The model under review builds one solid part; all positions refer to its coordinate system, in mm. A direction names the side the tool comes from. Give positions to 0.01 mm unless a question says otherwise; leave off trailing zeros. Order: outer loops, then holes, each group sorted by start corner. A loop starts at its lowest first (then second) coordinate and runs counter-clockwise, first axis right, second up. Notation, with made-up numbers: (19, 28.5) -> (34, 28.5) arc R30 ccw to (34, 52.5) -> close; hole circle Ø7 at (61.25, 61). An arc over 180 degrees is marked (long way). Answer as a JSON object with one key per item and string values. Group by question number.
from build123d import *

# Parameters (mm, degrees)
F0_R      = 55
F1_DEPTH  = 4
F2_R      = 22.1
F3_DEPTH  = 2
F4_R      = 25.3
F4_R_2    = 22.1
F5_DEPTH  = 1.5
F6_R      = 25.3
F6_R_2    = 23.5
F7_DEPTH  = 1.5
F8_DEPTH  = 0.2
F9_R      = 28
F9_R_2    = 25.3
F10_DEPTH = 1
F11_R     = 5
F12_DEPTH = 25
F14_DEPTH = 1
F15_R     = 1.45
F16_DEPTH = 25
F17_R     = 1.45
F18_DEPTH = 25


with BuildPart() as f1:
    # F0 (on Top) → F1 (new body)
    with BuildSketch(Plane.XY):
        Circle(F0_R)
    extrude(amount=F1_DEPTH)

    # F2 (on face) → F3 (cut)
    with BuildSketch(Plane.XY.offset(4)):
        with Locations((27, 0)):
            Circle(F2_R)
    extrude(amount=-F3_DEPTH, mode=Mode.SUBTRACT)

    # F4 (on face) → F5 (cut)
    with BuildSketch(Plane.XY.offset(4)):
        with Locations((27, 0)):
            Circle(F4_R)
        with Locations((27, 0)):
            Circle(F4_R_2, mode=Mode.SUBTRACT)
    extrude(amount=-F5_DEPTH, mode=Mode.SUBTRACT)

    # F6 (on face) → F7 (cut)
    with BuildSketch(Plane.XY.offset(2.5)):
        with Locations((27, 0)):
            Circle(F6_R)
        with Locations((27, 0)):
            Circle(F6_R_2, mode=Mode.SUBTRACT)
    extrude(amount=-F7_DEPTH, mode=Mode.SUBTRACT)

    # F8 (cut): a face of the model
    f8_faces = [f1.faces().sort_by_distance(p)[0] for p in [
        (4.1646803743, 0, 2.5),
    ]]
    extrude(f8_faces, amount=-F8_DEPTH, mode=Mode.SUBTRACT)

    # F9 (on face) → F10 (join)
    with BuildSketch(Plane.XY.offset(4)):
        with Locations((27, 0)):
            Circle(F9_R)
        with Locations((27, 0)):
            Circle(F9_R_2, mode=Mode.SUBTRACT)
    extrude(amount=F10_DEPTH)

    # F11 (on face) → F12 (cut)
    with BuildSketch(Plane.XY.offset(2)):
        with Locations((27, 0)):
            Circle(F11_R)
    extrude(amount=-F12_DEPTH, mode=Mode.SUBTRACT)

    # F13 (on face) → F14 (join)
    with BuildSketch(Plane.XY.offset(4)):
        with BuildLine():
            ThreePointArc((10.8848586854, -22.8976466129), (7.2010101268, -19.7989898732), (4.1023533871, -16.1151413146))
            ThreePointArc((4.1023533871, -16.1151413146), (2.9583694397, -24.0416305603), (10.8848586854, -22.8976466129))
        make_face()
        with BuildLine():
            ThreePointArc((10.8848586854, 22.8976466129), (2.9583694397, 24.0416305603), (4.1023533871, 16.1151413146))
            ThreePointArc((4.1023533871, 16.1151413146), (7.2010101268, 19.7989898732), (10.8848586854, 22.8976466129))
        make_face()
        with BuildLine():
            ThreePointArc((49.8976466129, -16.1151413146), (46.7989898732, -19.7989898732), (43.1151413146, -22.8976466129))
            ThreePointArc((43.1151413146, -22.8976466129), (45.5447053375, -25.105329645), (48.8197581332, -25.3304404978))
            ThreePointArc((48.8197581332, -25.3304404978), (50.4964850216, -21.7969034605), (51.917853321, -18.1531404043))
            ThreePointArc((51.917853321, -18.1531404043), (51.0570972643, -16.9860974117), (49.8976466129, -16.1151413146))
        make_face()
        with BuildLine():
            ThreePointArc((48.8197581332, 25.3304404978), (45.5447053375, 25.105329645), (43.1151413146, 22.8976466129))
            ThreePointArc((43.1151413146, 22.8976466129), (46.7989898732, 19.7989898732), (49.8976466129, 16.1151413146))
            ThreePointArc((49.8976466129, 16.1151413146), (51.0570972643, 16.9860974117), (51.917853321, 18.1531404043))
            ThreePointArc((51.917853321, 18.1531404043), (50.4964850216, 21.7969034605), (48.8197581332, 25.3304404978))
        make_face()
    extrude(amount=F14_DEPTH)

    # F15 (on face) → F16 (cut)
    with BuildSketch(Plane.XY.offset(5)):
        with Locations((6.4939033456, 20.5060966544)):
            Circle(F15_R)
        with Locations((47.5060966544, 20.5060966544)):
            Circle(F15_R)
        with Locations((47.5060966544, -20.5060966544)):
            Circle(F15_R)
        with Locations((6.4939033456, -20.5060966544)):
            Circle(F15_R)
    extrude(amount=-F16_DEPTH, mode=Mode.SUBTRACT)

    # F17 (on face) → F18 (cut)
    with BuildSketch(Plane.XY.offset(4)):
        with Locations((0, 45)):
            Circle(F17_R)
        with Locations((-45, 0)):
            Circle(F17_R)
        with Locations((0, -45)):
            Circle(F17_R)
    extrude(amount=-F18_DEPTH, mode=Mode.SUBTRACT)


solid = f1.part
1. Take a section at B-B on x = 27. Give the boundary of the cut face in (y, z).
2. Take a section at A-A on y = -45. Give the boundary of the cut face in (x, z).
3. Take a section at C-C on y = -10. Give the boundary of the cut face in (x, z), plus the area to 3 significant figures.
4. For probe 1 along Y at (x, z) = (28, 1.25); probe 2 along Y at (x, z) = (47, 4.5); probe 3 along Z at (x, y) = (37, 36), list the stretches that pass through material, from the lowest coordinate up. Write a range as [from, to].
5. Machinability: for faces 1 (the cylindrical face through (26.8, -28, 4.5)), 2 (the flat face through (11, -16, 2.3)), 3 (the cylindrical face through (6.18, -21.92, 2.54)), which of the approach directions +Z, -Z, +X, -X, +Y, -Y give a long, thin tool a straight path to every point of the face, cutting with its end or side? Answer none if there is none.
6. Take a section at D-D on x = -48. Give the boundary of the cut face in (y, z).
7. Draft analysis for pull direction X (two halves, no side actions). For faces 4 (the cylindrical face through (55, -0.2, 4.5)), 5 (the cylindrical face through (45.502, -25.087, 4.493)), 6 (the cylindrical face through (-1, 0.2, 4.5)), state which applies: pulls with the +X half, pulls with the -X half, needs draft (parallel to the pull), parting line crosses it, or undercut.
8. For pin 1 (4.5 mm diameter, centred on x = 47.51, y = -20.51, fed in from -Z); pin 2 (3 mm diameter, centred on x = -38.5, z = 2.5, fed in from +Y); pin 3 (2 mm diameter, centred on y = 4.5, z = 1.5, fed in from -X); pin 4 (6 mm diameter, centred on x = -25, y = -16, fed in from +Z), all flat-tipped, find the tip position at first contact; note any pin that passes through.
Checks:
{
 "1": {"outline": "(-47.92, 0) -> (-5, 0) -> (-5, 2) -> (-22.1, 2) -> (-22.1, 2.3) -> (-23.5, 2.3) -> (-23.5, 1) -> (-25.3, 1) -> (-25.3, 5) -> (-28, 5) -> (-28, 4) -> (-47.92, 4) -> close; (5, 0) -> (47.92, 0) -> (47.92, 4) -> (28, 4) -> (28, 5) -> (25.3, 5) -> (25.3, 1) -> (23.5, 1) -> (23.5, 2.3) -> (22.1, 2.3) -> (22.1, 2) -> (5, 2) -> close"},
 "2": {"outline": "(-31.62, 0) -> (-1.45, 0) -> (-1.45, 4) -> (-31.62, 4) -> close; (1.45, 0) -> (31.62, 0) -> (31.62, 4) -> (1.45, 4) -> close"},
 "3": {"outline": "(-54.08, 0) -> (54.08, 0) -> (54.08, 4) -> (53.15, 4) -> (53.15, 5) -> (50.24, 5) -> (50.24, 1) -> (48.27, 1) -> (48.27, 2.3) -> (46.71, 2.3) -> (46.71, 2) -> (7.29, 2) -> (7.29, 2.3) -> (5.73, 2.3) -> (5.73, 1) -> (3.76, 1) -> (3.76, 5) -> (0.85, 5) -> (0.85, 4) -> (-54.08, 4) -> close", "area": "343 mm2"},
 "4": {"probe 1": "y = [-47.34, -25.28], [-23.48, -4.9], [4.9, 23.48], [25.28, 47.34]", "probe 2": "y = [-25.48, -21.86], [-19.15, -15.49], [15.49, 19.15], [21.86, 25.48]", "probe 3": "z = [0, 4]"},
 "5": {"face 1": "+Z, -Y", "face 2": "+Z", "face 3": "+Z, -Z"},
 "6": {"outline": "(-26.85, 0) -> (26.85, 0) -> (26.85, 4) -> (-26.85, 4) -> close"},
 "7": {"face 4": "pulls with the +X half", "face 5": "undercut", "face 6": "pulls with the -X half"},
 "8": {"pin 1": "stops at z = 0", "pin 2": "stops at y = 40.69", "pin 3": "stops at x = -54.89", "pin 4": "stops at z = 4"}
}
